The model under review builds one solid part; all positions refer to its coordinate system, in mm. Face numbers are marked on the shaded views. Round coordinates to 2 decimals unless told otherwise and drop trailing zeros. Order: outer loops, then holes, each group sorted by start corner. A loop starts at its lowest first (then second) coordinate and runs counter-clockwise, first axis right, second up.
1) Consider section A-A (y = 4). Give the boundary of the cut face in (x, z), then the cut area to 3 significant figures.
2) Clearance check with a flat-ended pin moving along its axis: P1, Ø1.8, axis at x = 13, z = 4, coming from the -Y side. State where the tip first meets the part, or that it passes through.
3) Mouldability with a two-part tool opening along X and no side actions: class the marked faces 1, 2, 3 and 4 as pulls with the +X half, pulls with the -X half, needs draft (parallel to the pull), parting line crosses it, or undercut.
4) Consider section D-D (z = 6). Give the boundary of the cut face in (x, y), then the cut area to 3 significant figures.
5) Consider section C-C (x = 13). Give the boundary of the cut face in (y, z), then the cut area to 3 significant figures.
6) Consider section B-B (z = 3). Give the boundary of the cut face in (x, y).
7) To check wall thickness, follow L1, parallel to X at y = 5.75, z = 4; L2, parallel to Y at x = 26, z = 6; L3, parallel to X at y = 4.25, z = 6.5. State the ranges of each line that lie inside material, in increasing order.
from build123d import *

# Parameters (mm, degrees)
SKETCH_1_W          = 34
SKETCH_1_H          = 8
EXTRUDE_1_DEPTH     = 8
SKETCH_2_R          = 1.5
CUT_EXTRUDE_1_DEPTH = 36.832945734
SKETCH_3_R          = 1.5
CUT_EXTRUDE_2_DEPTH = 36.832945734


with BuildPart() as part:
    # 草图1 → 凸台-拉伸1 (new body)
    with BuildSketch(Plane.XY):
        with Locations((17, 4)):
            Rectangle(SKETCH_1_W, SKETCH_1_H)
    extrude(amount=EXTRUDE_1_DEPTH)

    # 草图2 → 切除-拉伸1 (cut, through all)
    with BuildSketch(Plane.XY.offset(8)):
        with Locations((8, 4)):
            Circle(SKETCH_2_R)
        with Locations((26, 4)):
            Circle(SKETCH_2_R)
    extrude(amount=-CUT_EXTRUDE_1_DEPTH, mode=Mode.SUBTRACT)

    # 草图3 → 切除-拉伸2 (cut, through all)
    with BuildSketch(Plane(origin=(0, 8, 0), x_dir=(1, 0, 0), z_dir=(0, 1, 0))):
        with Locations(Location((13, -4, 0), (0, 0, 270))):
            Circle(SKETCH_3_R)
        with Locations(Location((21, -4, 0), (0, 0, 270))):
            Circle(SKETCH_3_R)
    extrude(amount=-CUT_EXTRUDE_2_DEPTH, mode=Mode.SUBTRACT)


solid = part.part
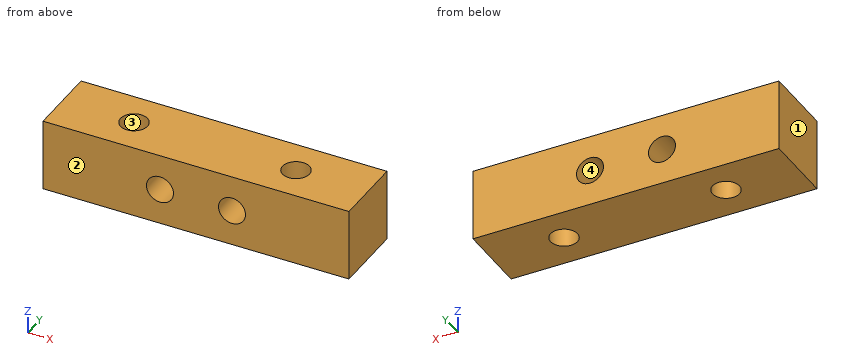
Answer below:
1. outline: (0, 0) - (6.5, 0) - (6.5, 8) - (0, 8) - close; (9.5, 0) - (24.5, 0) - (24.5, 8) - (9.5, 8) - close; (27.5, 0) - (34, 0) - (34, 8) - (27.5, 8) - close; hole circle Ø3 at (13, 4); hole circle Ø3 at (21, 4)
1. area: 210 mm2
2. P1: passes through
3. face 1: pulls with the -X half
3. face 2: needs draft
3. face 3: undercut
3. face 4: undercut
4. outline: (0, 0) - (34, 0) - (34, 8) - (0, 8) - close; hole circle Ø3 at (8, 4); hole circle Ø3 at (26, 4)
4. area: 258 mm2
5. outline: (0, 0) - (8, 0) - (8, 2.5) - (0, 2.5) - close; (0, 5.5) - (8, 5.5) - (8, 8) - (0, 8) - close
5. area: 40.0 mm2
6. outline: (0, 0) - (11.88, 0) - (11.88, 8) - (0, 8) - close; (14.12, 0) - (19.88, 0) - (19.88, 8) - (14.12, 8) - close; (22.12, 0) - (34, 0) - (34, 8) - (22.12, 8) - close; hole circle Ø3 at (8, 4); hole circle Ø3 at (26, 4)
7. L1: x = 0 to 11.5, 14.5 to 19.5, 22.5 to 34
7. L2: y = 0 to 2.5, 5.5 to 8
7. L3: x = 0 to 6.52, 9.48 to 24.52, 27.48 to 34
